from build123d import *

# Parameters (mm, degrees)
SCHIZZO1_R                   = 1.5
ESTRUSIONE_ESTRUSIONE1_DEPTH = 4


with BuildPart() as part:
    # Schizzo1 → Estrusione-Estrusione1 (new body)
    with BuildSketch(Plane.XY):
        with BuildLine():
            Line((0, -15), (49.434299833, -15))
            ThreePointArc((49.434299833, -15), (56.874189574, -6.552349937), (47.554189972, -0.239477504))
            ThreePointArc((47.554189972, -0.239477504), (27.787162994, 0.02445935), (10.90104019, 10.30375285))
            ThreePointArc((10.90104019, 10.30375285), (-13.775998925, 5.934800218), (0, -15))
        make_face()
        Circle(SCHIZZO1_R, mode=Mode.SUBTRACT)
        with Locations((49.434299833, -7.5)):
            Circle(SCHIZZO1_R, mode=Mode.SUBTRACT)
    extrude(amount=ESTRUSIONE_ESTRUSIONE1_DEPTH)


solid = part.part
Work out the finished part from the listing and answer in its coordinate system (mm). Give positions to 0.01 mm unless a question says otherwise; leave off trailing zeros. Write each loop counter-clockwise with the first axis right and the second up, starting at its lowest first coordinate (ties: lowest second). Pieces come first, ordered by that corner, then holes. Notation, with made-up numbers: M 23,8 L 61,8 A33 cw 61,39 Z; hole C 56,63.5 d4. An arc over 180 degrees is marked long. Answer as CSV lines item,"result".
Q1. A cutting plane is placed at C-C on x = 9.5. Write down the section's boundary in (y, z), plus the area to 3 significant figures.
A:
outline,"M -15,0 L 11.61,0 L 11.61,4 L -15,4 Z"
area,"106 mm²"
Q2. A cutting plane is placed at D-D on y = 4. Write down the section's boundary in (x, z).
A:
outline,"M -14.46,0 L 18.71,0 L 18.71,4 L -14.46,4 Z"
Q3. The mould has two halves that part along X. Classify faces 1 (the flat face through (12, -3, 0)), 2 (the cylindrical face through (-13.61, 6.31, 1.97)), 3 (the cylindrical face through (28.057, -0.052, 1.972)), 4 (the cylindrical face through (-1.5, 0.07, 1.97)): +X half, -X half, draft (parallel to the pull), parting line (faces both ways), or undercut.
A:
face 1,"draft"
face 2,"parting line"
face 3,"undercut"
face 4,"undercut"
Q4. A cutting plane is placed at A-A on y = -7.5. Write down the section's boundary in (x, z), plus the area to 3 significant figures.
A:
outline,"M -12.99,0 L 47.93,0 L 47.93,4 L -12.99,4 Z; M 50.93,0 L 56.93,0 L 56.93,4 L 50.93,4 Z"
area,"268 mm²"
Q5. Find the intervals of material crossed by probe 1 along Y at (x, z) = (0, 2.3); probe 2 along Y at (x, z) = (49.5, 0.7); probe 3 along X at (y, z) = (12.5, 3.45), in increasing order. Write a range as [from, to].
A:
probe 1,"y = [-15, -1.5], [1.5, 15]"
probe 2,"y = [-15, -9], [-6, 0]"
probe 3,"x = [-8.29, 8.29]"
Q6. A cutting plane is placed at B-B on z = 2.05. Write down the section's boundary in (x, y).
A:
outline,"M 0,-15 L 49.43,-15 A7.5 ccw long 47.55,-0.24 A37.5 cw 10.9,10.3 A15 ccw long Z; hole C 0,0 d3; hole C 49.43,-7.5 d3"
